The drawing under review shows one solid part. Ordinate dimensions are in mm from its lowest x, y, z. A direction names the side the tool comes from. Give positions to 0.01 mm unless a question says otherwise; leave off trailing zeros. Write each loop counter-clockwise with the first axis right and the second up, starting at its lowest first coordinate (ties: lowest second). Pieces come first, ordered by that corner, then holes.
Q1. We need section A-A (y = 18.5). Write out the cut boundary in (x, z).
Q2. We need section B-B (x = 7). Write out the cut boundary in (y, z).
Q3. For line 1 (Y direction, x = 15, z = 48.3) (3 decimals); line 2 (Z direction, x = 12.25, y = 12.5); line 3 (X direction, y = 16, z = 32), list the stretches that pass through material, from the lowest coordinate up.
Q4. Machinability: for the marked faces 1 and 2, which of the approach directions +Z, -Z, +X, -X, +Y, -Y give a long, thin tool a straight path to every point of the face, cutting with its end or side? Answer none if there is none.
Q5. Mouldability with a two-part tool opening along X and no side actions: class the marked faces 3, 4, 5 and 6 as released by +X, released by -X, zero draft, split by the parting line, or undercut.
Q6. We need section C-C (z = 20). Write out the cut boundary in (x, y).
Q7. We need section D-D (y = 28). Write out the cut boundary in (x, z).
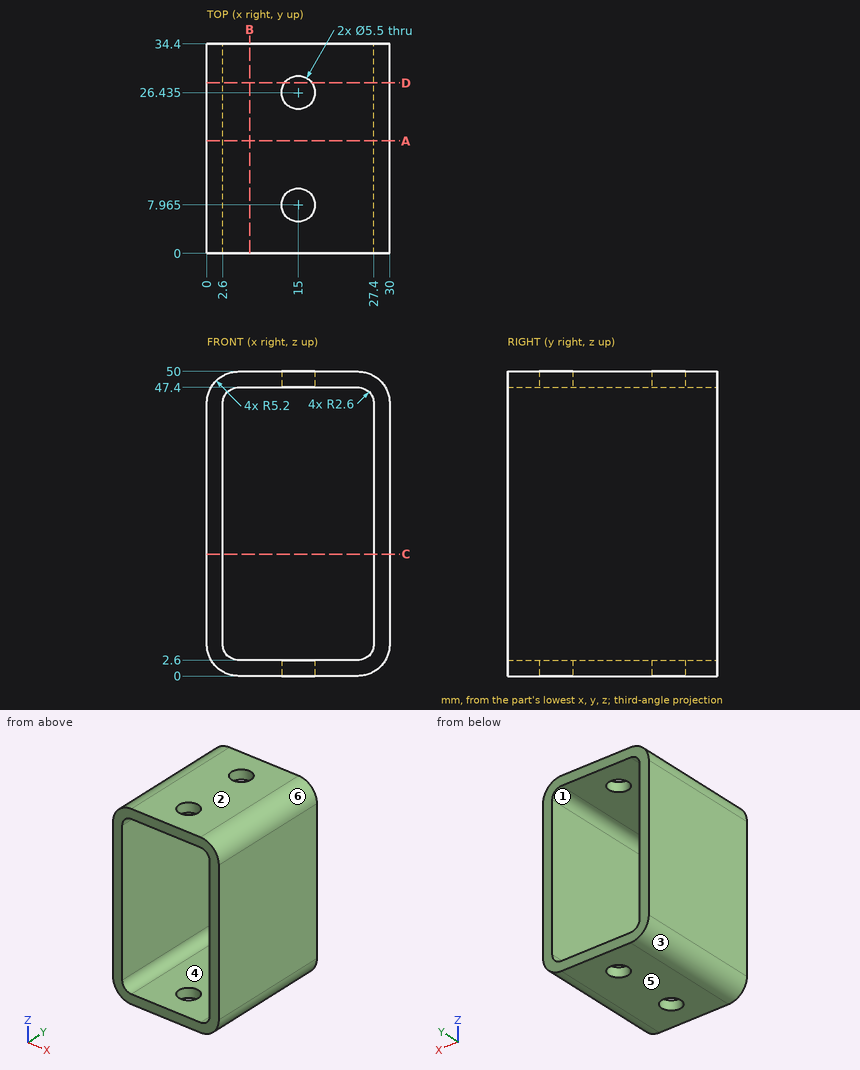
Computed:
1. outline: (0, 5.2) arc R5.2 ccw to (5.2, 0) - (24.8, 0) arc R5.2 ccw to (30, 5.2) - (30, 44.8) arc R5.2 ccw to (24.8, 50) - (5.2, 50) arc R5.2 ccw to (0, 44.8) - close; hole (2.6, 5.2) arc R2.6 ccw to (5.2, 2.6) - (24.8, 2.6) arc R2.6 ccw to (27.4, 5.2) - (27.4, 44.8) arc R2.6 ccw to (24.8, 47.4) - (5.2, 47.4) arc R2.6 ccw to (2.6, 44.8) - close
2. outline: (0, 0) - (34.4, 0) - (34.4, 2.6) - (0, 2.6) - close; (0, 47.4) - (34.4, 47.4) - (34.4, 50) - (0, 50) - close
3. line 1: y = 0 to 5.215, 10.715 to 23.685, 29.185 to 34.4
3. line 2: z = 0 to 2.6, 47.4 to 50
3. line 3: x = 0 to 2.6, 27.4 to 30
4. face 1: +Y, -Y
4. face 2: +Z, +X, -X, +Y, -Y
5. face 3: released by -X
5. face 4: undercut
5. face 5: zero draft
5. face 6: released by +X
6. outline: (0, 0) - (2.6, 0) - (2.6, 34.4) - (0, 34.4) - close; (27.4, 0) - (30, 0) - (30, 34.4) - (27.4, 34.4) - close
7. outline: (0, 5.2) arc R5.2 ccw to (5.2, 0) - (12.74, 0) - (12.74, 2.6) - (5.2, 2.6) arc R2.6 cw to (2.6, 5.2) - (2.6, 44.8) arc R2.6 cw to (5.2, 47.4) - (12.74, 47.4) - (12.74, 50) - (5.2, 50) arc R5.2 ccw to (0, 44.8) - close; (17.26, 0) - (24.8, 0) arc R5.2 ccw to (30, 5.2) - (30, 44.8) arc R5.2 ccw to (24.8, 50) - (17.26, 50) - (17.26, 47.4) - (24.8, 47.4) arc R2.6 cw to (27.4, 44.8) - (27.4, 5.2) arc R2.6 cw to (24.8, 2.6) - (17.26, 2.6) - close
